```python
from build123d import *

# Parameters (mm, degrees)
SKETCH1_W           = 129.9464
SKETCH1_H           = 83.9724
BOSS_EXTRUDE1_DEPTH = 5.7912
SKETCH2_W           = 9.872133334
SKETCH2_H           = 5.7912
CUT_EXTRUDE1_DEPTH  = 6.7912
SKETCH3_W           = 5.7912
SKETCH3_H           = 27.9908
CUT_EXTRUDE2_DEPTH  = 6.7912
SKETCH4_W           = 13.7668
SKETCH4_H           = 2.6035
CUT_EXTRUDE3_DEPTH  = 6.7912
SKETCH6_W           = 2.0828
SKETCH6_H           = 6.1722
CUT_EXTRUDE5_DEPTH  = 6.7912
SKETCH7_W           = 106.1212
SKETCH7_H           = 82.55
BOSS_EXTRUDE2_DEPTH = 5.7912
SKETCH8_W           = 43.315466666
SKETCH8_H           = 5.7912
CUT_EXTRUDE6_DEPTH  = 6.7912
SKETCH12_W          = 5.7912
SKETCH12_H          = 27.516666666
CUT_EXTRUDE9_DEPTH  = 6.7912
SKETCH13_W          = 13.7668
SKETCH13_H          = 2.6035
CUT_EXTRUDE10_DEPTH = 6.7912
SKETCH14_W          = 2.0828
SKETCH14_H          = 6.1722
CUT_EXTRUDE11_DEPTH = 6.7912
SKETCH15_W          = 35.373733334
SKETCH15_H          = 5.7912
CUT_EXTRUDE12_DEPTH = 6.7912


with BuildPart() as part:
    # Sketch1 → Boss-Extrude1 (new body)
    with BuildSketch(Plane.XY):
        Rectangle(SKETCH1_W, SKETCH1_H)
    extrude(amount=BOSS_EXTRUDE1_DEPTH)

    # Sketch2 → Cut-Extrude1 (cut, through all)
    with BuildSketch(Plane.XY.offset(5.7912)):
        with Locations((-50.165, 39.0906)):
            Rectangle(SKETCH2_W, SKETCH2_H)
    extrude(amount=-CUT_EXTRUDE1_DEPTH, mode=Mode.SUBTRACT)

    # Sketch3 → Cut-Extrude2 (cut, through all)
    with BuildSketch(Plane.XY.offset(5.7912)):
        with Locations((-62.0776, 0)):
            Rectangle(SKETCH3_W, SKETCH3_H)
        with Locations((62.0776, 0)):
            Rectangle(SKETCH3_W, SKETCH3_H)
    extrude(amount=-CUT_EXTRUDE2_DEPTH, mode=Mode.SUBTRACT)

    # Sketch4 → Cut-Extrude3 (cut, through all)
    with BuildSketch(Plane.XY.offset(5.7912)):
        with Locations((52.2986, 0)):
            Rectangle(SKETCH4_W, SKETCH4_H)
    extrude(amount=-CUT_EXTRUDE3_DEPTH, mode=Mode.SUBTRACT)

    # Sketch6 → Cut-Extrude5 (cut, through all)
    with BuildSketch(Plane.XY.offset(5.7912)):
        with Locations((55.3212, 0)):
            Rectangle(SKETCH6_W, SKETCH6_H)
    extrude(amount=-CUT_EXTRUDE5_DEPTH, mode=Mode.SUBTRACT)

    # Sketch7 → Boss-Extrude2 (add)
    with BuildSketch(Plane.XY.offset(5.7912)):
        with Locations((11.9126, 83.2612)):
            Rectangle(SKETCH7_W, SKETCH7_H)
    extrude(amount=-BOSS_EXTRUDE2_DEPTH)

    # Sketch8 → Cut-Extrude6 (cut, through all)
    with BuildSketch(Plane.XY.offset(5.7912)):
        with Locations((0, -39.0906)):
            Rectangle(SKETCH8_W, SKETCH8_H)
    extrude(amount=-CUT_EXTRUDE6_DEPTH, mode=Mode.SUBTRACT)

    # Sketch12 → Cut-Extrude9 (cut, through all)
    with BuildSketch(Plane.XY.offset(5.7912)):
        with Locations((62.0776, 83.2612)):
            Rectangle(SKETCH12_W, SKETCH12_H)
        with Locations((-38.2524, 83.2612)):
            Rectangle(SKETCH12_W, SKETCH12_H)
    extrude(amount=-CUT_EXTRUDE9_DEPTH, mode=Mode.SUBTRACT)

    # Sketch13 → Cut-Extrude10 (cut, through all)
    with BuildSketch(Plane.XY.offset(5.7912)):
        with Locations((52.2986, 83.2612)):
            Rectangle(SKETCH13_W, SKETCH13_H)
    extrude(amount=-CUT_EXTRUDE10_DEPTH, mode=Mode.SUBTRACT)

    # Sketch14 → Cut-Extrude11 (cut, through all)
    with BuildSketch(Plane.XY.offset(5.7912)):
        with Locations((51.2572, 83.2612)):
            Rectangle(SKETCH14_W, SKETCH14_H)
    extrude(amount=-CUT_EXTRUDE11_DEPTH, mode=Mode.SUBTRACT)

    # Sketch15 → Cut-Extrude12 (cut, through all)
    with BuildSketch(Plane.XY.offset(5.7912)):
        with Locations((11.9126, 121.6406)):
            Rectangle(SKETCH15_W, SKETCH15_H)
    extrude(amount=-CUT_EXTRUDE12_DEPTH, mode=Mode.SUBTRACT)


solid = part.part
```
Verification items for the finished model (mm, model axes). A direction names the side the tool comes from. Round coordinates to 2 decimals unless told otherwise and drop trailing zeros. Write each loop counter-clockwise with the first axis right and the second up, starting at its lowest first coordinate (ties: lowest second). Pieces come first, ordered by that corner, then holes.
1. Gauge pin test, flat ends, axial feed: P1, Ø2, axis at y = 81, z = 3.5, coming from the +X side; P2, Ø2, axis at y = 81, z = 3, coming from the -X side; P3, Ø1.7, axis at x = -60.5, z = 3, coming from the +Y side; P4, Ø1.5, axis at x = 4, y = -24, coming from the -Z side. Record the tip position at first contact, or that the pin passes through.
2. Draft check along X on faces 4 (the flat face through (-45.229, 39, 3)), 5 (the flat face through (29.599, 122, 3)), 6 (the flat face through (59.182, 76, 3)), 7 (the flat face through (62, 69.503, 3)). Enter one of: +X half, -X half, draft (parallel to the pull), parting line (faces both ways), or undercut.
3. Section check B-B on x = 24. Enter the section's corners in (y, z) (3 decimals).
4. Section check A-A on y = 12. Enter the section's corners in (x, z), plus the area to 3 significant figures.
5. Access from +Z, -Z, +X, -X, +Y, -Y to the whole of each face (thin tool, end or side, straight path). Record for faces 1 (the flat face through (-59.182, 0, 3)), 2 (the flat face through (12, 118.745, 3)), 3 (the flat face through (56, 84.563, 3)).
6. Scan lines: L1, parallel to Y at x = 56, z = 1.85; L2, parallel to X at y = 40.5, z = 0.35; L3, parallel to X at y = 85, z = 1.2. Record each from-to range of solid material in increasing order.
Answer:
1. P1: stops at x = 59.18
1. P2: stops at x = -35.36
1. P3: stops at y = 41.99
1. P4: stops at z = 0
2. face 4: undercut
2. face 5: undercut
2. face 6: +X half
2. face 7: draft
3. outline: (-41.986, 0) - (118.745, 0) - (118.745, 5.791) - (-41.986, 5.791) - close
4. outline: (-59.18, 0) - (59.18, 0) - (59.18, 5.79) - (-59.18, 5.79) - close
4. area: 685 mm2
5. face 1: +Z, -Z, -X
5. face 2: +Z, -Z, +Y
5. face 3: +Z, -Z, +X
6. L1: y = -41.99 to -3.09, 3.09 to 81.96, 84.56 to 124.54
6. L2: x = -64.97 to -55.1, -45.23 to 64.97
6. L3: x = -35.36 to 50.22, 52.3 to 59.18
